Build history of the part. All positions in model axes, mm. A direction names the side the tool comes from. Give positions to 0.01 mm unless a question says otherwise; leave off trailing zeros. Loops run counter-clockwise (first coordinate to the right, second up) from the corner with the lowest first, then second, coordinate; pieces in that order, holes last. Notation, with made-up numbers: M -17.5,-38.5 L 4.5,-38.5 A17 cw 4.5,-25.5 Z; hole C 25,10 d5. An arc over 180 degrees is marked long. Answer as a JSON object with one key per item and string values. Group by question number.
1. Slice it at A-A (x = 5). List the corners of the cut face in (y, z).
2. 3-axis set-ups, long thin cutter, end or side, ignore diameter. For faces 5 (the face through (20.405, -9, -15)), 6 (the face through (6.882, 13.078, -17.226)), 7 (the face through (5, -18.97, -12)), 8 (the face through (-30, 31.015, -3)): which of +Z, -Z, +X, -X, +Y, -Y reach the whole face in a straight line?
3. Slice it at C-C (x = 28). List the corners of the cut face in (y, z).
4. Drill centre lines: line 1 along Z through (x, y) = (-1.5, 33.5); line 2 along Y through (x, z) = (-0.5, -6.75); line 3 along Z through (x, y) = (-30, 6.5). Where is each one in solid material? Low to high. Write a range as [from, to].
5. Mould opens along X. For faces 1 (the face through (5.195, 28.977, -14.486)), 2 (the face through (-39.623, 28.132, -2.465)), 3 (the face through (5, 51.03, -12)), 4 (the face through (25.358, -7, -2)) say: released by +X, released by -X, zero draft, split by the parting line, or undercut.
6. Drop flat-ended pins along their axis: pin 1 Ø11 at (y, z) = (-11, -12) entering from -X; pin 2 Ø10 at (y, z) = (8.5, -14.5) entering from +X; pin 3 Ø5 at (x, y) = (51.6, 27.51) entering from -Z; pin 4 Ø10 at (x, y) = (-2.5, 41.5) entering from +Z. Give the stop position or say it passes through.
7. Slice it at B-B (x = -13). List the corners of the cut face in (y, z).
from build123d import *

# Parameters (mm, degrees)
F0_W      = 40.765519
F0_H      = 73.471674
F1_DEPTH  = 5
F2_R      = 3.5
F3_DEPTH  = 14
F4_W      = 35
F4_H      = 50.010137
F5_DEPTH  = 8.5
F6_W      = 100
F6_H      = 24.910029
F7_DEPTH  = 5
F8_R      = 1.85
F9_DEPTH  = 25.4
F10_R     = 12.94909
F11_DEPTH = 2


with BuildPart() as f1:
    # F0 (on Top) → F1 (new body)
    with BuildSketch(Plane.XY):
        with Locations((4.975075, 16.320152)):
            Rectangle(F0_W, F0_H)
    extrude(amount=-F1_DEPTH)

    # F2 (on face) → F3 (join)
    with BuildSketch(Plane(origin=(0, 0, -5), x_dir=(1, 0, 0), z_dir=(0, 0, -1))):
        with BuildLine():
            Line((20.405405, 18.970378), (-10.405405, 18.970378))
            Line((-10.405405, 18.970378), (-10.405405, -7.227108))
            ThreePointArc((-10.405405, -7.227108), (-1.55183, -16.080683), (-10.405405, -24.934258))
            Line((-10.405405, -24.934258), (-10.405405, -51.029622))
            Line((-10.405405, -51.029622), (20.405405, -51.029622))
            Line((20.405405, -51.029622), (20.405405, -24.883203))
            ThreePointArc((20.405405, -24.883203), (11.551825, -16.029622), (20.405405, -7.176042))
            Line((20.405405, -7.176042), (20.405405, 18.970378))
        make_face()
        with Locations((5, -16.029622)):
            Circle(F2_R, mode=Mode.SUBTRACT)
    extrude(amount=F3_DEPTH)

    # F4 (on face) → F5 (cut)
    with BuildSketch(Plane(origin=(0, 0, -5), x_dir=(1, 0, 0), z_dir=(0, 0, -1))):
        with Locations((2.905405, -15.991903)):
            Rectangle(F4_W, F4_H)
    extrude(amount=F5_DEPTH, mode=Mode.SUBTRACT)

    # F6 (on face) → F7 (join)
    with BuildSketch(Plane(origin=(0, 0, -5), x_dir=(1, 0, 0), z_dir=(0, 0, -1))):
        with Locations((5.092296, -18.559826)):
            Rectangle(F6_W, F6_H)
    extrude(amount=-F7_DEPTH)

    # F8 (on face) → F9 (cut)
    with BuildSketch(Plane.XY):
        with Locations((-41.387634, 27.575926)):
            Circle(F8_R)
        with Locations((51.599746, 27.514396)):
            Circle(F8_R)
        with Locations((-41.413683, 9.564399)):
            Circle(F8_R)
        with Locations((51.624972, 9.70294)):
            Circle(F8_R)
    extrude(amount=-F9_DEPTH, mode=Mode.SUBTRACT)

    # F10 (on face) → F11 (cut)
    with BuildSketch(Plane.XY.offset(-13.5)):
        with Locations((5, 16.029622)):
            Circle(F10_R)
    extrude(amount=-F11_DEPTH, mode=Mode.SUBTRACT)


solid = f1.part
Established:
{
 "1": {"outline": "M -20.42,-5 L -18.97,-5 L -18.97,-19 L 12.53,-19 L 12.53,-15.5 L 3.08,-15.5 L 3.08,-13.5 L -9.01,-13.5 L -9.01,-5 L 41,-5 L 41,-13.5 L 28.98,-13.5 L 28.98,-15.5 L 19.53,-15.5 L 19.53,-19 L 51.03,-19 L 51.03,-5 L 53.06,-5 L 53.06,0 L -20.42,0 Z"},
 "2": {"face 5": "-Z, +X, +Y, -Y", "face 6": "-Z", "face 7": "-Z, +X, -X, -Y", "face 8": "+Z, -Z, -X, +Y"},
 "3": {"outline": "M 6.1,-5 L 31.01,-5 L 31.01,0 L 6.1,0 Z"},
 "4": {"line 1": "z = [-19, -13.5], [-5, 0]", "line 2": "y = [-18.97, -9.01], [41, 51.03]", "line 3": "z = [-5, 0]"},
 "5": {"face 1": "undercut", "face 2": "undercut", "face 3": "zero draft", "face 4": "released by +X"},
 "6": {"pin 1": "stops at x = -10.41", "pin 2": "stops at x = 20.41", "pin 3": "stops at z = -5", "pin 4": "stops at z = 0"},
 "7": {"outline": "M -20.42,-5 L 53.06,-5 L 53.06,0 L -20.42,0 Z"}
}
